```python
from build123d import *

# Parameters (mm, degrees)
EXTRUDE_630_DEPTH           = 2
CUT_EXTRUDE_1091_DEPTH      = 311.882614503
CUT_EXTRUDE_1091_DEPTH_BACK = 311.882614503
SKETCH_5_R                  = 1.5
CUT_EXTRUDE_1860_DEPTH      = 311.882614503
CUT_EXTRUDE_1860_DEPTH_BACK = 311.882614503
SKETCH_10_R                 = 1.5
CUT_EXTRUDE_2028_DEPTH      = 311.882614503
CUT_EXTRUDE_2028_DEPTH_BACK = 311.882614503
SKETCH_11_R                 = 2
CUT_EXTRUDE_2382_DEPTH      = 311.882614503
CUT_EXTRUDE_2382_DEPTH_BACK = 311.882614503
SKETCH_12_W                 = 5
SKETCH_12_H                 = 19
SKETCH_12_H_2               = 37
CUT_EXTRUDE_2536_DEPTH      = 311.882614503
CUT_EXTRUDE_2536_DEPTH_BACK = 311.882614503
SKETCH_13_R                 = 1.5


with BuildPart() as part:
    # 草图1 → Extrude 630 (new, symmetric)
    with BuildSketch(Plane(origin=(0, 0, 0), x_dir=(1, 0, 0), z_dir=(0, 1, 0))):
        Polygon((290, -63), (290, 63), (242, 63), (242, 89), (201, 89), (201, 112), (101, 112), (101, 89), (60, 89), (60, 68), (5, 68), (5, -68), (60, -68), (60, -89), (101, -89), (101, -98), (201, -98), (201, -89), (242, -89), (242, -63), align=None)
    extrude(amount=EXTRUDE_630_DEPTH, both=True)

    # 草图5 → Cut-Extrude 1091 (cut, two sides: drawn at the far end of the back side and taken through both)
    with BuildSketch(Plane(origin=(0, 0, 0), x_dir=(1, 0, 0), z_dir=(0, 1, 0)).offset(-CUT_EXTRUDE_1091_DEPTH_BACK)):
        with Locations(Location((65.5, 84, 0), (0, 0, 270))):
            Circle(SKETCH_5_R)
        with Locations(Location((95.5, 84, 0), (0, 0, 270))):
            Circle(SKETCH_5_R)
        with Locations(Location((65.5, 61, 0), (0, 0, 270))):
            Circle(SKETCH_5_R)
        with Locations(Location((95.5, 61, 0), (0, 0, 270))):
            Circle(SKETCH_5_R)
        with Locations(Location((206.5, 61, 0), (0, 0, 270))):
            Circle(SKETCH_5_R)
        with Locations(Location((206.5, 84, 0), (0, 0, 270))):
            Circle(SKETCH_5_R)
        with Locations(Location((236.5, 61, 0), (0, 0, 270))):
            Circle(SKETCH_5_R)
        with Locations(Location((236.5, 83, 0), (0, 0, 270))):
            Circle(SKETCH_5_R)
        with Locations(Location((236.5, -61, 0), (0, 0, 90))):
            Circle(SKETCH_5_R)
        with Locations(Location((206.5, -61, 0), (0, 0, 90))):
            Circle(SKETCH_5_R)
        with Locations(Location((236.5, -83, 0), (0, 0, 90))):
            Circle(SKETCH_5_R)
        with Locations(Location((206.5, -84, 0), (0, 0, 90))):
            Circle(SKETCH_5_R)
        with Locations(Location((95.5, -61, 0), (0, 0, 90))):
            Circle(SKETCH_5_R)
        with Locations(Location((95.5, -84, 0), (0, 0, 90))):
            Circle(SKETCH_5_R)
        with Locations(Location((65.5, -61, 0), (0, 0, 90))):
            Circle(SKETCH_5_R)
        with Locations(Location((65.5, -84, 0), (0, 0, 90))):
            Circle(SKETCH_5_R)
    extrude(amount=CUT_EXTRUDE_1091_DEPTH + CUT_EXTRUDE_1091_DEPTH_BACK, mode=Mode.SUBTRACT)

    # 草图10 → Cut-Extrude 1860 (cut, two sides: drawn at the far end of the back side and taken through both)
    with BuildSketch(Plane(origin=(0, 0, 0), x_dir=(1, 0, 0), z_dir=(0, 1, 0)).offset(-CUT_EXTRUDE_1860_DEPTH_BACK)):
        with Locations(Location((106, 108.159987948, 0), (0, 0, 270))):
            Circle(SKETCH_10_R)
        with Locations(Location((196, 108.159987948, 0), (0, 0, 270))):
            Circle(SKETCH_10_R)
        with Locations(Location((106, -33.340012052, 0), (0, 0, 270))):
            Circle(SKETCH_10_R)
        with Locations(Location((196, -33.340012052, 0), (0, 0, 270))):
            Circle(SKETCH_10_R)
    extrude(amount=CUT_EXTRUDE_1860_DEPTH + CUT_EXTRUDE_1860_DEPTH_BACK, mode=Mode.SUBTRACT)

    # 草图11 → Cut-Extrude 2028 (cut, two sides: drawn at the far end of the back side and taken through both)
    with BuildSketch(Plane(origin=(0, 0, 0), x_dir=(1, 0, 0), z_dir=(0, 1, 0)).offset(-CUT_EXTRUDE_2028_DEPTH_BACK)):
        with Locations(Location((91, 20, 0), (0, 0, 270))):
            Circle(SKETCH_11_R)
        with Locations(Location((91, -20, 0), (0, 0, 270))):
            Circle(SKETCH_11_R)
        with Locations(Location((211, 20, 0), (0, 0, 270))):
            Circle(SKETCH_11_R)
        with Locations(Location((211, -20, 0), (0, 0, 270))):
            Circle(SKETCH_11_R)
    extrude(amount=CUT_EXTRUDE_2028_DEPTH + CUT_EXTRUDE_2028_DEPTH_BACK, mode=Mode.SUBTRACT)

    # 草图12 → Cut-Extrude 2382 (cut, two sides: drawn at the far end of the back side and taken through both)
    with BuildSketch(Plane(origin=(0, 0, 0), x_dir=(1, 0, 0), z_dir=(0, 1, 0)).offset(-CUT_EXTRUDE_2382_DEPTH_BACK)):
        with Locations((245.321540625, 22.5)):
            Rectangle(SKETCH_12_W, SKETCH_12_H)
        with Locations((245.321540625, -22.5)):
            Rectangle(SKETCH_12_W, SKETCH_12_H)
        with Locations((225.321540625, 0)):
            Rectangle(SKETCH_12_W, SKETCH_12_H_2)
    extrude(amount=CUT_EXTRUDE_2382_DEPTH + CUT_EXTRUDE_2382_DEPTH_BACK, mode=Mode.SUBTRACT)

    # 草图13 → Cut-Extrude 2536 (cut, two sides: drawn at the far end of the back side and taken through both)
    with BuildSketch(Plane(origin=(0, 0, 0), x_dir=(1, 0, 0), z_dir=(0, 1, 0)).offset(-CUT_EXTRUDE_2536_DEPTH_BACK)):
        with Locations(Location((282.881144326, 33, 0), (0, 0, 270))):
            Circle(SKETCH_13_R)
        with Locations(Location((282.881144326, -33, 0), (0, 0, 270))):
            Circle(SKETCH_13_R)
    extrude(amount=CUT_EXTRUDE_2536_DEPTH + CUT_EXTRUDE_2536_DEPTH_BACK, mode=Mode.SUBTRACT)


solid = part.part
```
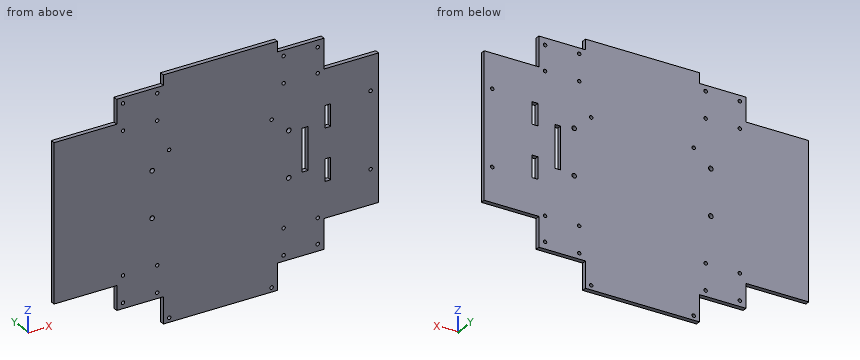
Geometry: final body of the model. Coordinates: model frame, mm. Coordinates: 2 decimals unless noted, no trailing zeros. Write each loop counter-clockwise with the first axis right and the second up, starting at its lowest first coordinate (ties: lowest second). Pieces come first, ordered by that corner, then holes. Notation, with made-up numbers: M -3,77.5 L 6,77.5 A12 ccw 6,88.5 Z; hole C 25.25,54.25 d8. An arc over 180 degrees is marked long. Use CSV: the item, a comma, the result in double quotes. Start each with the question number.
1. Cut plane A-A on x = 218. Return the cut outline in (y, z).
2. Ray query, probe 1 along X at (y, z) = (-0.45, -16); probe 2 along Z at (x, y) = (65.5, -0.3); probe 3 along Z at (x, y) = (106, -0.8). Return the intervals inside material, ascending.
3. First-contact query: P1, Ø2.5, axis at x = 282.88, z = -33, coming from the +Y side; P2, Ø4, axis at x = 206.5, z = -84, coming from the -Y side; P3, Ø1.2, axis at x = 25.5, y = 0.5, coming from the +Z side. Flat tips, straight axial feed; report the tip coordinate or a pass-through.
4. Cut plane B-B on z = 72.5. Return the cut outline in (x, y).
5. Cut plane C-C on y = 0.05. Count the separate pieces of the cut face and the enclosed holes in it, plus the area to 3 significant figures.
Entries:
1,outline,"M -2,-89 L 2,-89 L 2,89 L -2,89 Z"
2,probe 1,"5 to 222.82, 227.82 to 242.82, 247.82 to 290"
2,probe 2,"-89 to -85.5, -82.5 to -62.5, -59.5 to 59.5, 62.5 to 82.5, 85.5 to 89"
2,probe 3,"-112 to -109.66, -106.66 to 31.84, 34.84 to 98"
3,P1,"through"
3,P2,"y = -2"
3,P3,"z = 68"
4,outline,"M 60,-2 L 242,-2 L 242,2 L 60,2 Z"
5,separate pieces,"1"
5,enclosed holes,"29"
5,area,"48,500 mm²"
